Input: dimensioned drawing with shaded views. Units: mm. Origin: part minimum x, y, z. A direction names the side the tool comes from. Round coordinates to 2 decimals unless told otherwise and drop trailing zeros. Loops run counter-clockwise (first coordinate to the right, second up) from the corner with the lowest first, then second, coordinate; pieces in that order, holes last. Notation, with made-up numbers: (82, 1) - (87, 1) arc R25 cw to (87, 28) - close; hole circle Ø11 at (4, 25.25). An arc over 180 degrees is marked (long way). One line per question, with ' | ' between items.
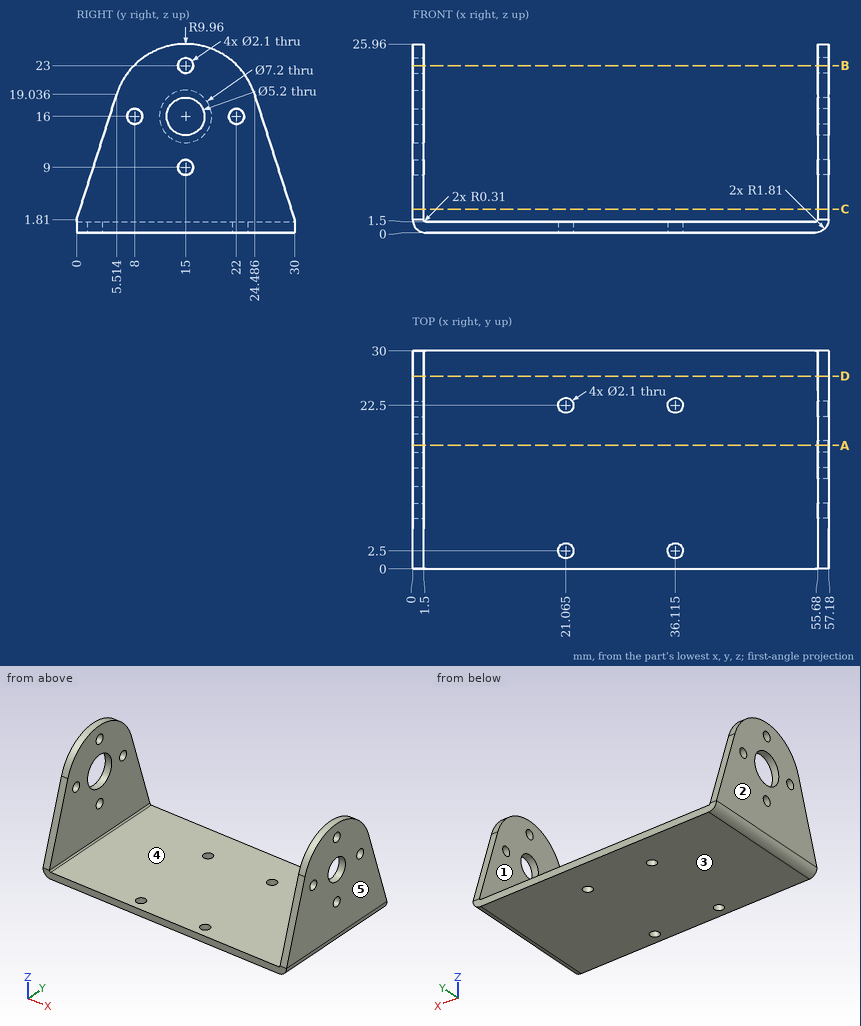
1. Section query A-A, the plane y = 17. Return loops of the section in (x, z).
Worked out:
outline: (0, 1.81) arc R1.81 ccw to (1.81, 0) - (55.37, 0) arc R1.81 ccw to (57.18, 1.81) - (57.18, 14.34) - (55.68, 14.34) - (55.68, 1.81) arc R0.31 cw to (55.37, 1.5) - (1.81, 1.5) arc R0.31 cw to (1.5, 1.81) - (1.5, 13.01) - (0, 13.01) - close; (0, 18.99) - (1.5, 18.99) - (1.5, 25.76) - (0, 25.76) - close; (55.68, 17.66) - (57.18, 17.66) - (57.18, 25.76) - (55.68, 25.76) - close
2. Contact query for flat-ended pins moving along their axis: P1, Ø3, axis at x = 32, y = 6, coming from the -Z side; P2, Ø15, axis at x = 34.5, y = 8, coming from the +Z side; P3, Ø6.5, axis at y = 15, z = 16, coming from the -X side. Output: stop coordinate, or through.
Worked out:
P1: stops at z = 0 | P2: stops at z = 1.5 | P3: stops at x = 55.68
3. Mould query, pull axis X, two halves, no side actions, for the marked faces 1, 2 and 3. Classes: released by +X, released by -X, zero draft, split by the parting line, or undercut.
Worked out:
face 1: undercut | face 2: released by -X | face 3: zero draft
4. Access query for the marked faces 4 and 5. Directions: +Z, -Z, +X, -X, +Y, -Y. A direction counts if a zero-diameter tool reaches every point of the face in a straight line with its end or side. Return the directions, or none.
Worked out:
face 4: +Z, +Y, -Y | face 5: +Z, -Z, +X, +Y, -Y
5. Material intervals for probe 1 along Y at (x, z) = (0.5, 16); probe 2 along X at (y, z) = (24, 12.25); probe 3 along X at (y, z) = (2.5, 0.55) (1 decimal), sorted ascending.
Worked out:
probe 1: y = 4.54 to 6.95, 9.05 to 11.4, 18.6 to 20.95, 23.05 to 25.46 | probe 2: x = 0 to 1.5, 55.68 to 57.18 | probe 3: x = 0.5 to 20, 22.1 to 35.1, 37.2 to 56.7
6. Section query D-D, the plane y = 26.5. Return loops of the section in (x, z) (1 decimal), plus the area to 3 significant figures.
Worked out:
outline: (0, 1.8) arc R1.8 ccw to (1.8, 0) - (55.4, 0) arc R1.8 ccw to (57.2, 1.8) - (57.2, 12.7) - (55.7, 12.7) - (55.7, 1.8) arc R0.3 cw to (55.4, 1.5) - (1.8, 1.5) arc R0.3 cw to (1.5, 1.8) - (1.5, 12.7) - (0, 12.7) - close | area: 118 mm2
7. Section query B-B, the plane z = 23. Give the number of separate pieces and of enclosed holes in the cut face.
Worked out:
separate pieces: 4 | enclosed holes: 0
8. Section query C-C, the plane z = 3.25. Return loops of the section in (x, y).
Worked out:
outline: (0, 0.46) - (1.5, 0.46) - (1.5, 29.54) - (0, 29.54) - close; (55.68, 0.46) - (57.18, 0.46) - (57.18, 29.54) - (55.68, 29.54) - close
